Work out the finished part from the listing and answer in its coordinate system (mm). A direction names the side the tool comes from. Round coordinates to 2 decimals unless told otherwise and drop trailing zeros. Order: outer loops, then holes, each group sorted by start corner. A loop starts at its lowest first (then second) coordinate and runs counter-clockwise, first axis right, second up. Notation, with made-up numbers: (-20, -19) - (9, -19) arc R10 cw to (9, -5) - close; hole circle Ø1 at (3.25, -3). An arc over 180 degrees is marked (long way). Put each result on its own line as item: value.
```python
from build123d import *

# Parameters (mm, degrees)
SKETCH1_R           = 175
SKETCH1_R_2         = 55
BOSS_EXTRUDE1_DEPTH = 12.5
SKETCH2_W           = 40
SKETCH2_H           = 6
SKETCH2_W_2         = 6
SKETCH2_H_2         = 40
CUT_EXTRUDE2_DEPTH  = 249.746859277
SKETCH3_R           = 5
CUT_EXTRUDE3_DEPTH  = 249.746859277


with BuildPart() as part:
    # Sketch1 → Boss-Extrude1 (new, symmetric)
    with BuildSketch(Plane(origin=(0, 0, 0), x_dir=(1, 0, 0), z_dir=(0, 1, 0))):
        with Locations(Location((0, 0, 0), (0, 0, 270))):
            Circle(SKETCH1_R)
        with Locations(Location((0, 0, 0), (0, 0, 270))):
            Circle(SKETCH1_R_2, mode=Mode.SUBTRACT)
    extrude(amount=BOSS_EXTRUDE1_DEPTH, both=True)

    # Sketch2 → Cut-Extrude2 (cut, through all)
    with BuildSketch(Plane(origin=(0, 12.5, 0), x_dir=(1, 0, 0), z_dir=(0, 1, 0))):
        with Locations((0, 170)):
            Rectangle(SKETCH2_W, SKETCH2_H)
        Polygon((103.944696834, 132.228968082), (132.228968082, 103.944696834), (136.471608769, 108.187337522), (108.187337522, 136.471608769), align=None)
        with Locations((170, 0)):
            Rectangle(SKETCH2_W_2, SKETCH2_H_2)
        Polygon((132.228968082, -103.944696834), (103.944696834, -132.228968082), (108.187337522, -136.471608769), (136.471608769, -108.187337522), align=None)
        with Locations((0, -170)):
            Rectangle(SKETCH2_W, SKETCH2_H)
        Polygon((-103.944696834, -132.228968082), (-132.228968082, -103.944696834), (-136.471608769, -108.187337522), (-108.187337522, -136.471608769), align=None)
        with Locations((-170, 0)):
            Rectangle(SKETCH2_W_2, SKETCH2_H_2)
        Polygon((-132.228968082, 103.944696834), (-103.944696834, 132.228968082), (-108.187337522, 136.471608769), (-136.471608769, 108.187337522), align=None)
    extrude(amount=-CUT_EXTRUDE2_DEPTH, mode=Mode.SUBTRACT)

    # Sketch3 → Cut-Extrude3 (cut, through all)
    with BuildSketch(Plane(origin=(0, 12.5, 0), x_dir=(1, 0, 0), z_dir=(0, 1, 0))):
        with Locations(Location((-90, 90, 0), (0, 0, 270))):
            Circle(SKETCH3_R)
        with Locations(Location((90, 90, 0), (0, 0, 90))):
            Circle(SKETCH3_R)
        with Locations(Location((90, -90, 0), (0, 0, 270))):
            Circle(SKETCH3_R)
        with Locations(Location((-90, -90, 0), (0, 0, 90))):
            Circle(SKETCH3_R)
    extrude(amount=-CUT_EXTRUDE3_DEPTH, mode=Mode.SUBTRACT)


solid = part.part
```
1) Given pin 1 Ø12 at (y, z) = (6.5, -52) entering from +X; pin 2 Ø5 at (y, z) = (7, -4) entering from +X; pin 3 Ø3 at (y, z) = (-6, -13) entering from -X, each flat-ended and moving along its own axis, determine where each tip first touches the part or whether it passes through.
Findings below:
pin 1: stops at x = 168.85
pin 2: stops at x = 174.99
pin 3: stops at x = -174.62
2) For faces 1 (the flat face through (41, 12.5, -41)), 2 (the flat face through (0, 0, 173)), determine the directions among +Z, -Z, +X, -X, +Y, -Y from which every point of the face is accessible in a straight line to the end or side of a thin tool.
Findings below:
face 1: +Z, -Z, +X, -X, +Y
face 2: +Y, -Y
3) Straight lines are drawn through the part: L1, parallel to X at y = -4.5, z = -90; L2, parallel to X at y = -4, z = 126; L3, parallel to Z at x = 12.5, y = -10.75. For each, find the intervals that lie inside material, in ascending order. Write a range as from..to.
Findings below:
L1: x = -150.08..-95, -85..85, 95..150.08
L2: x = -121.45..-118.66, -110.17..110.17, 118.66..121.45
L3: z = -174.55..-173, -167..-53.56, 53.56..167, 173..174.55
4) For a pull along Z with two mould halves and no side action, classify faces 3 (the cylindrical face through (173.51, 0.18, -22.78)), 4 (the flat face through (41, -12.5, -41)), 5 (the flat face through (-173, 0, 0)) as pulls with the +Z half, pulls with the -Z half, needs draft (parallel to the pull), parting line crosses it, or undercut.
Findings below:
face 3: parting line crosses it
face 4: needs draft
face 5: undercut
5) A cutting plane is placed at B-B on z = 0. Write down the section's boundary in (x, y), then the cut area to 3 significant figures.
Findings below:
outline: (-175, -12.5) - (-173, -12.5) - (-173, 12.5) - (-175, 12.5) - close; (-167, -12.5) - (-55, -12.5) - (-55, 12.5) - (-167, 12.5) - close; (55, -12.5) - (167, -12.5) - (167, 12.5) - (55, 12.5) - close; (173, -12.5) - (175, -12.5) - (175, 12.5) - (173, 12.5) - close
area: 5,700 mm2
6) A cutting plane is placed at D-D on z = -90. Write down the section's boundary in (x, y), then the cut area to 3 significant figures.
Findings below:
outline: (-150.08, -12.5) - (-95, -12.5) - (-95, 12.5) - (-150.08, 12.5) - close; (-85, -12.5) - (85, -12.5) - (85, 12.5) - (-85, 12.5) - close; (95, -12.5) - (150.08, -12.5) - (150.08, 12.5) - (95, 12.5) - close
area: 7,000 mm2
7) A cutting plane is placed at A-A on x = 0. Write down the section's boundary in (y, z).
Findings below:
outline: (-12.5, -175) - (12.5, -175) - (12.5, -173) - (-12.5, -173) - close; (-12.5, -167) - (12.5, -167) - (12.5, -55) - (-12.5, -55) - close; (-12.5, 55) - (12.5, 55) - (12.5, 167) - (-12.5, 167) - close; (-12.5, 173) - (12.5, 173) - (12.5, 175) - (-12.5, 175) - close
8) A cutting plane is placed at C-C on x = -90. Write down the section's boundary in (y, z).
Findings below:
outline: (-12.5, -150.08) - (12.5, -150.08) - (12.5, -95) - (-12.5, -95) - close; (-12.5, -85) - (12.5, -85) - (12.5, 85) - (-12.5, 85) - close; (-12.5, 95) - (12.5, 95) - (12.5, 150.08) - (-12.5, 150.08) - close
